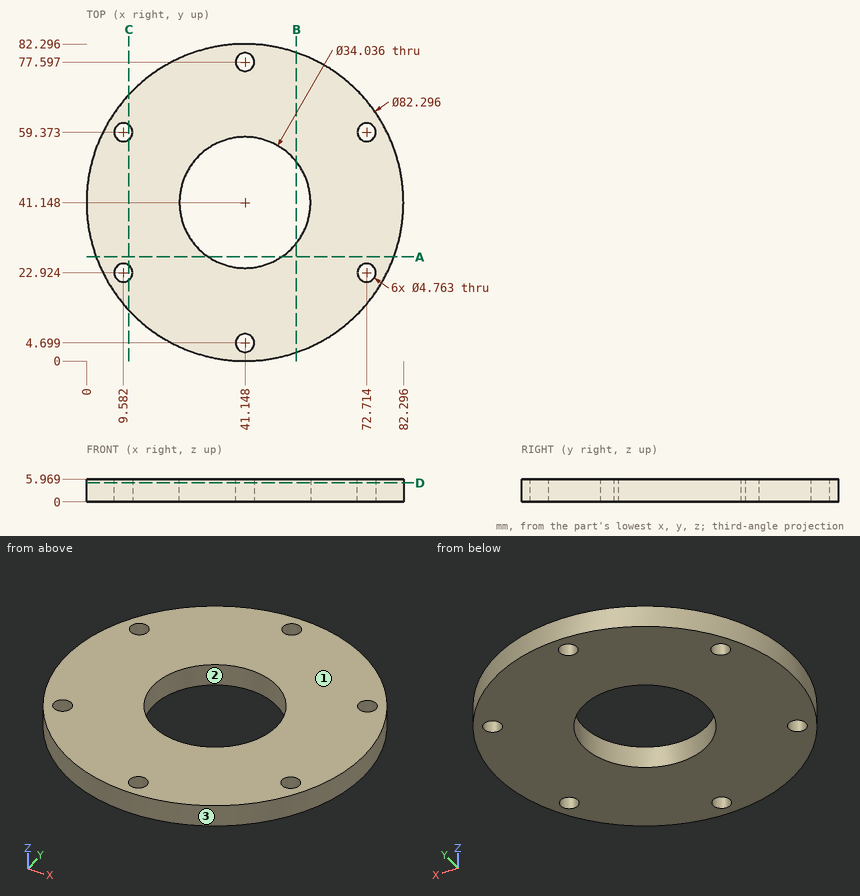
The figure shows three views and two pictorial views of one solid part (mm, origin at its lowest corner). Answer the questions. Round coordinates to 2 decimals unless told otherwise and drop trailing zeros. Write each loop counter-clockwise with the first axis right and the second up, starting at its lowest first coordinate (ties: lowest second). Pieces come first, ordered by that corner, then holes. Notation, with made-up numbers: (47.5, 62.5) -> (101.5, 62.5) arc R31 cw to (101.5, 101.5) -> close; hole circle Ø7 at (-29, -39). An arc over 180 degrees is marked (long way). Write each question's results on one line, items separated by ' | '.
Q1. Straight lines are drawn through the part: line 1 along X through (y, z) = (21.5, 5.55) (1 decimal); line 2 along X through (y, z) = (40.5, 3.9) (1 decimal); line 3 along Y through (x, z) = (48, 4.1) (1 decimal). For each, find the intervals that lie inside material, in ascending order. Write a range as [from, to].
Data:
line 1: [5, 7.7], [11.5, 70.8], [74.6, 77.3] | line 2: [0, 24.1], [58.2, 82.3] | line 3: [0.6, 25.6], [56.7, 81.7]
Q2. Section B-B, the plane x = 54.5 is taken. Write down the section's boundary in (y, z), then the cut area to 3 significant figures.
Data:
outline: (2.23, 0) -> (30.6, 0) -> (30.6, 5.97) -> (2.23, 5.97) -> close; (51.7, 0) -> (80.07, 0) -> (80.07, 5.97) -> (51.7, 5.97) -> close | area: 339 mm^2
Q3. Section C-C, the plane x = 11 is taken. Write down the section's boundary in (y, z) (1 decimal).
Data:
outline: (13.1, 0) -> (21, 0) -> (21, 6) -> (13.1, 6) -> close; (24.8, 0) -> (57.5, 0) -> (57.5, 6) -> (24.8, 6) -> close; (61.3, 0) -> (69.2, 0) -> (69.2, 6) -> (61.3, 6) -> close
Q4. Section A-A, the plane y = 27 is taken. Write down the section's boundary in (x, z) (1 decimal).
Data:
outline: (2.5, 0) -> (31.7, 0) -> (31.7, 6) -> (2.5, 6) -> close; (50.6, 0) -> (79.8, 0) -> (79.8, 6) -> (50.6, 6) -> close
Q5. Determine the mould class of the marked faces 1, 2 and 3 for opening direction Y: released by +Y, released by -Y, zero draft, split by the parting line, or undercut.
Data:
face 1: zero draft | face 2: undercut | face 3: split by the parting line
Q6. Section D-D, the plane z = 4.95 is taken. Write down the section's boundary in (x, y) (1 decimal), then the cut area to 3 significant figures.
Data:
outline: circle Ø82.3 at (41.1, 41.1); hole circle Ø4.8 at (9.6, 22.9); hole circle Ø4.8 at (9.6, 59.4); hole circle Ø34 at (41.1, 41.1); hole circle Ø4.8 at (41.1, 4.7); hole circle Ø4.8 at (41.1, 77.6); hole circle Ø4.8 at (72.7, 22.9); hole circle Ø4.8 at (72.7, 59.4) | area: 4,300 mm^2
Q7. Flat-ended cylindrical pins translate along their axes: P1, Ø1.5, axis at x = 41.5, y = 24.5, coming from the -Z side; P2, Ø1.5, axis at y = 68.5, z = 1, coming from the +X side; P3, Ø3, axis at y = 26.5, z = 3.5, coming from the +X side. Find the tip coordinate at first contact, or state that the pin passes through.
Data:
P1: z = 0 | P2: x = 72.54 | P3: x = 80.14
